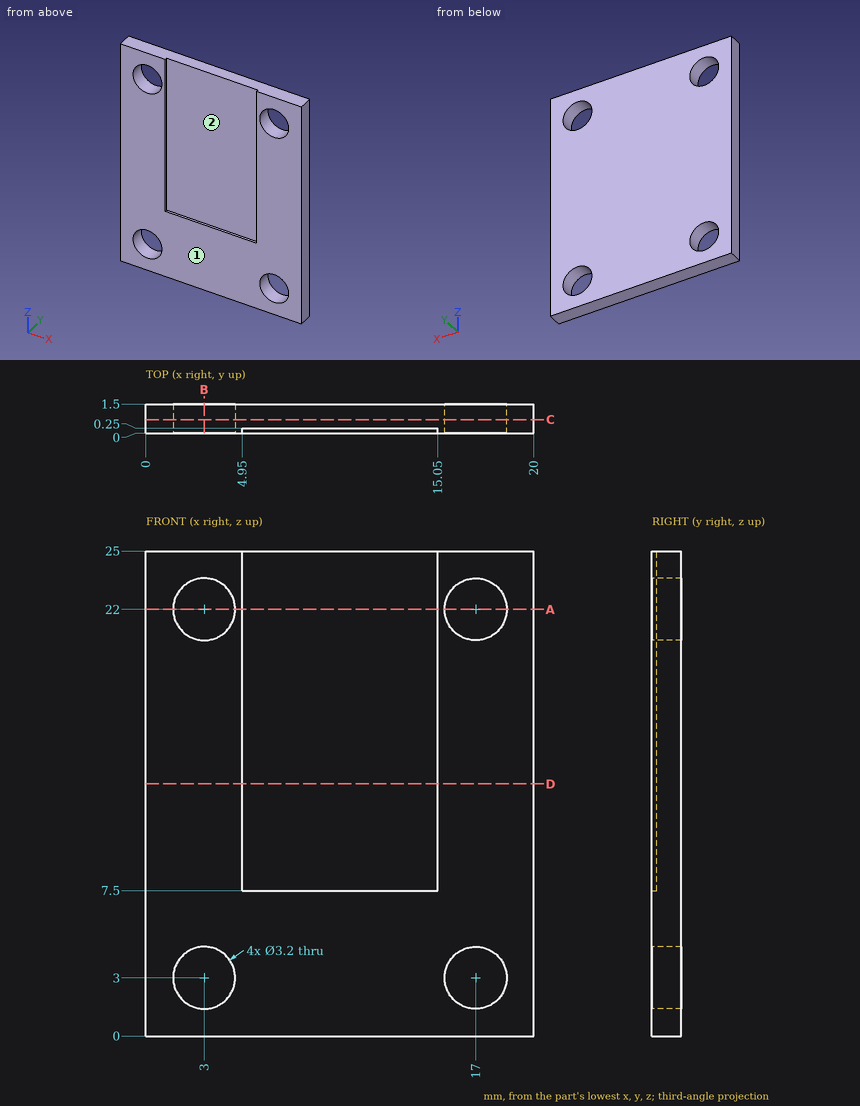
Can you work these out from the drawing? Everything is in mm from the part's minimum corner. A direction names the side the tool comes from. Coordinates: 2 decimals unless noted, no trailing zeros. Loops run counter-clockwise (first coordinate to the right, second up) from the corner with the lowest first, then second, coordinate; pieces in that order, holes last.
1) Imagine slicing it at B-B on x = 3. List the corners of the cut face in (y, z) for me, plus the area to 3 significant figures.
2) I need wall thicknesses on probe 1 along Z at (x, y) = (17, 0.4); probe 2 along X at (y, z) = (1.15, 22); probe 3 along X at (y, z) = (0.1, 23). Which ranges of each line are inside material? Lowest first, please.
3) Which directions (+Z, -Z, +X, -X, +Y, -Y) give clear straight access to the entire face, cutting with the end or side of a thin tool? Please do the marked faces 1 and 2.
4) Imagine slicing it at A-A on z = 22. List the corners of the cut face in (x, y) for me, plus the area to 3 significant figures.
5) Imagine slicing it at D-D on z = 13. List the corners of the cut face in (x, y) for me, plus the area to 3 significant figures.
6) Imagine slicing it at C-C on y = 0.7. List the corners of the cut face in (x, z) for me.
Completed:
1. outline: (0, 0) - (1.5, 0) - (1.5, 1.4) - (0, 1.4) - close; (0, 4.6) - (1.5, 4.6) - (1.5, 20.4) - (0, 20.4) - close; (0, 23.6) - (1.5, 23.6) - (1.5, 25) - (0, 25) - close
1. area: 27.9 mm2
2. probe 1: z = 0 to 1.4, 4.6 to 20.4, 23.6 to 25
2. probe 2: x = 0 to 1.4, 4.6 to 15.4, 18.6 to 20
2. probe 3: x = 0 to 1.75, 4.25 to 4.95, 15.05 to 15.75, 18.25 to 20
3. face 1: +Z, -Z, +X, -X, -Y
3. face 2: +Z, -Y
4. outline: (0, 0) - (1.4, 0) - (1.4, 1.5) - (0, 1.5) - close; (4.6, 0) - (4.95, 0) - (4.95, 0.25) - (15.05, 0.25) - (15.05, 0) - (15.4, 0) - (15.4, 1.5) - (4.6, 1.5) - close; (18.6, 0) - (20, 0) - (20, 1.5) - (18.6, 1.5) - close
4. area: 17.9 mm2
5. outline: (0, 0) - (4.95, 0) - (4.95, 0.25) - (15.05, 0.25) - (15.05, 0) - (20, 0) - (20, 1.5) - (0, 1.5) - close
5. area: 27.5 mm2
6. outline: (0, 0) - (20, 0) - (20, 25) - (0, 25) - close; hole circle Ø3.2 at (3, 3); hole circle Ø3.2 at (3, 22); hole circle Ø3.2 at (17, 3); hole circle Ø3.2 at (17, 22)
